For this review, use the dimensioned drawing (mm, ordinates from the lowest corner) and the shaded views. A direction names the side the tool comes from. Round coordinates to 2 decimals unless told otherwise and drop trailing zeros. Loops run counter-clockwise (first coordinate to the right, second up) from the corner with the lowest first, then second, coordinate; pieces in that order, holes last. Notation, with made-up numbers: (-1, 49) -> (43, 49) arc R35 cw to (43, 87) -> close; hole circle Ø5 at (87, -24.5). An arc over 180 degrees is marked (long way). Answer as CSV lines item,"result". Start each with the question number.
(1) To check wall thickness, follow line 1 (X direction, y = 17.5, z = 10); line 2 (X direction, y = 43.5, z = 10); line 3 (Y direction, x = 12, z = 13.25). State the ranges of each line that lie inside material, in increasing order. Write a range as from..to.
(2) Machinability: for the marked faces 1 and 2, which of the approach directions +Z, -Z, +X, -X, +Y, -Y give a long, thin tool a straight path to every point of the face, cutting with its end or side? Answer none if there is none.
(3) For P1, Ø10, axis at x = 10, z = 10, coming from the +Y side; P2, Ø6, axis at y = 26, z = 15.5, coming from the +X side; P3, Ø1.5, axis at x = 9.5, z = 8, coming from the -Y side; P4, Ø1, axis at x = 18, y = 39, coming from the -Z side (1 decimal), all flat-tipped, find the tip position at first contact; note any pin that passes through.
(4) Take a section at A-A, the plane y = 37.5. Write out the cut boundary in (x, z).
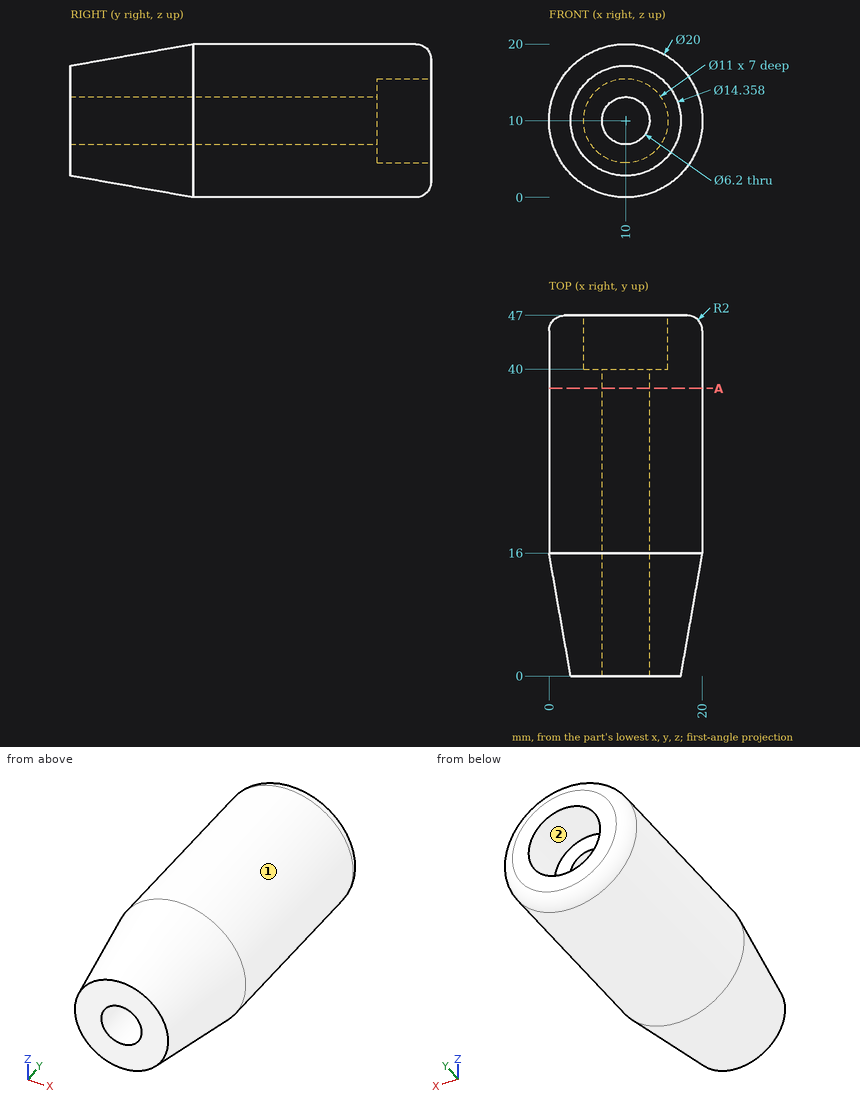
The answers:
1,line 1,"0..6.9, 13.1..20"
1,line 2,"0..4.5, 15.5..20"
1,line 3,"0..40"
2,face 1,"+Y, -Y"
2,face 2,"+Y"
3,P1,"y = 40"
3,P2,"x = 19.68"
3,P3,"through"
3,P4,"z = 3.4"
4,outline,"circle Ø20 at (10, 10); hole circle Ø6.2 at (10, 10)"
